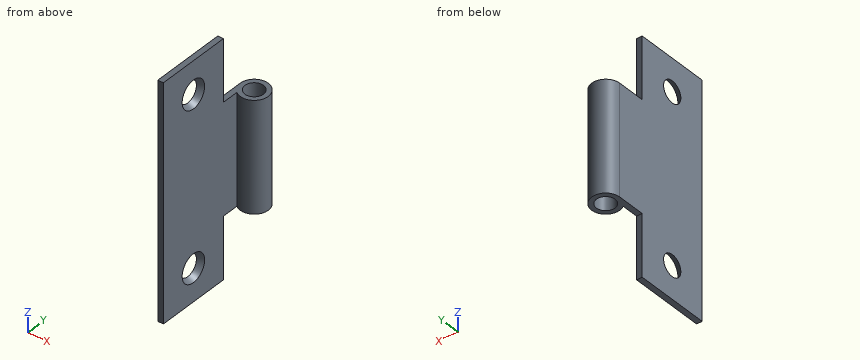
```python
from build123d import *

# Parameters (mm, degrees)
SKETCH_1_W          = 0.6
SKETCH_1_H          = 11
EXTRUDE_1_DEPTH     = 12.5
SKETCH_2_R          = 1.5
SKETCH_3_R          = 1
CUT_EXTRUDE_1_DEPTH = 29.111385594
SKETCH_10_W         = 7.870368163
SKETCH_10_H         = 6
CUT_EXTRUDE_4_DEPTH = 60
SKETCH_12_R         = 1.15
SKETCH_11_R         = 1.5


with BuildPart() as part:
    # 草图1 → 拉伸-薄壁1 (new, symmetric)
    with BuildSketch(Plane.XY):
        with Locations((0.3, 5.5)):
            Rectangle(SKETCH_1_W, SKETCH_1_H)
    extrude(amount=EXTRUDE_1_DEPTH, both=True)

    # 扫描1: sweep along a curve in space
    with BuildLine() as sweep_1_path:
        Line((0.6, 11, 12.5), (0.6, 11, -12.5))
    # 草图2 → 扫描1 (sweep)
    with BuildSketch(Plane.XY.offset(12.5)):
        with Locations((1.5, 11)):
            Circle(SKETCH_2_R)
    sweep(path=sweep_1_path.line)

    # 草图3 → 切除-拉伸1 (cut, through all)
    with BuildSketch(Plane.XY.offset(12.5)):
        with Locations((1.5, 11)):
            Circle(SKETCH_3_R)
    extrude(amount=-CUT_EXTRUDE_1_DEPTH, mode=Mode.SUBTRACT)

    # 草图10 → 切除-拉伸4 (cut, symmetric)
    with BuildSketch(Plane(origin=(0.6, 0, 0), x_dir=(0, 0, -1), z_dir=(1, 0, 0))):
        with Locations((-9.835184081, 11)):
            Rectangle(SKETCH_10_W, SKETCH_10_H)
        with Locations((9.835184081, 11)):
            Rectangle(SKETCH_10_W, SKETCH_10_H)
    extrude(amount=CUT_EXTRUDE_4_DEPTH, both=True, mode=Mode.SUBTRACT)

    # 草图12 → 切除-放样1 section 0
    with BuildSketch(Plane.ZY):
        with Locations((-9, 4)):
            Circle(SKETCH_12_R)
    # 草图11 → 切除-放样1 section 1
    with BuildSketch(Plane(origin=(0.6, 0, 0), x_dir=(0, 0, -1), z_dir=(1, 0, 0))):
        with Locations((9, 4)):
            Circle(SKETCH_11_R)
    loft_1 = loft(mode=Mode.SUBTRACT)

    # 镜向1: 切除-放样1 across plane
    add(loft_1.mirror(Plane.XY), mode=Mode.SUBTRACT)


solid = part.part
```
Source: CAD feature listing. Evaluate the final solid. Frame: model axes, mm. Round coordinates to 2 decimals unless told otherwise and drop trailing zeros. Order: outer loops, then holes, each group sorted by start corner. A loop starts at its lowest first (then second) coordinate and runs counter-clockwise, first axis right, second up. Notation, with made-up numbers: (67.5, 72) -> (75.5, 72) arc R18 ccw to (75.5, 80) -> close; hole circle Ø2 at (31, 45.25). An arc over 180 degrees is marked (long way). One line per item, written item: value. Start each with the question number.
Q1. Section query A-A (z = 9). Return the cut outline in (x, y).
Q2. Section query D-D (y = 4). Give the number of separate pieces and of enclosed holes in the cut face, plus the area to 3 significant figures.
Q3. Section query C-C (z = 2.5). Return the cut outline in (x, y), plus the area to 3 significant figures.
Q4. Pin query (flat end, axial travel): pin 1 (3 mm diameter, centred on y = 7, z = 7.5, fed in from +X); pin 2 (0.7 mm diameter, centred on x = 0.5, z = 9, fed in from +Y). Return the tip coordinate at first contact, or that it passes through.
Q5. Material intervals for probe 1 along Y at (x, z) = (1.5, 2.25); probe 2 along X at (y, z) = (8.25, 0.25); probe 3 along Y at (x, z) = (0.5, -10.75), sorted ascending.
Q6. Section query B-B (x = 1.5). Return the cut outline in (y, z).
Findings below:
1. outline: (0, 0) -> (0.6, 0) -> (0.6, 2.5) -> (0, 2.85) -> close; (0, 5.15) -> (0.6, 5.5) -> (0.6, 8) -> (0, 8) -> close
2. separate pieces: 3
2. enclosed holes: 0
2. area: 11.8 mm²
3. outline: (0, 0) -> (0.6, 0) -> (0.6, 9.8) arc R1.5 ccw (long way) to (0, 11) -> close; hole circle Ø2 at (1.5, 11)
3. area: 10.0 mm²
4. pin 1: x = 0.6
4. pin 2: y = 8
5. probe 1: 9.5 to 10, 12 to 12.5
5. probe 2: 0 to 0.6
5. probe 3: 0 to 8
6. outline: (9.5, -5.9) -> (10, -5.9) -> (10, 5.9) -> (9.5, 5.9) -> close; (12, -5.9) -> (12.5, -5.9) -> (12.5, 5.9) -> (12, 5.9) -> close
